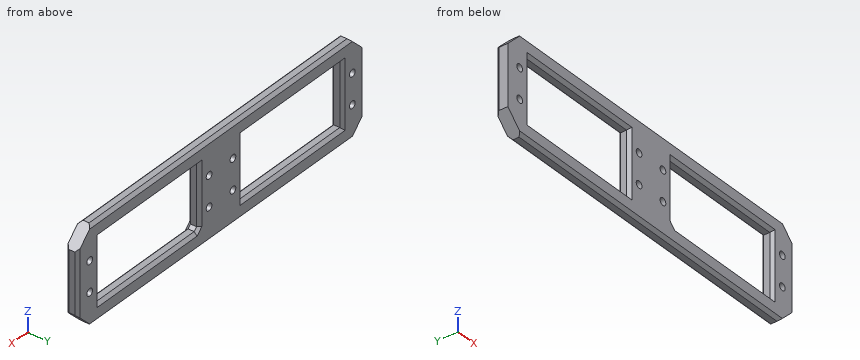
```python
from build123d import *

# Parameters (mm, degrees)
SKETCH1_W           = 120
SKETCH1_H           = 32
BOSS_EXTRUDE1_DEPTH = 4
SKETCH2_R           = 1.2
SKETCH2_W           = 42
SKETCH2_H           = 21
CUT_EXTRUDE1_DEPTH  = 4
CHAMFER1_SIZE       = 1
CUT_EXTRUDE2_DEPTH  = 10


with BuildPart() as part:
    # Sketch1 → Boss-Extrude1 (new body)
    with BuildSketch(Plane(origin=(0, 0, 0), x_dir=(1, 0, 0), z_dir=(0, 1, 0))):
        Rectangle(SKETCH1_W, SKETCH1_H)
    extrude(amount=BOSS_EXTRUDE1_DEPTH)

    # Sketch2 → Cut-Extrude1 (cut)
    with BuildSketch(Plane(origin=(0, 4, 0), x_dir=(1, 0, 0), z_dir=(0, 1, 0))):
        with Locations(Location((55, 5, 0), (0, 0, 270))):
            Circle(SKETCH2_R)
        with Locations(Location((55, -5, 0), (0, 0, 270))):
            Circle(SKETCH2_R)
        with Locations(Location((5, 5, 0), (0, 0, 270))):
            Circle(SKETCH2_R)
        with Locations(Location((5, -5, 0), (0, 0, 270))):
            Circle(SKETCH2_R)
        with Locations((30, 0)):
            Rectangle(SKETCH2_W, SKETCH2_H)
    cut_extrude1 = extrude(amount=-CUT_EXTRUDE1_DEPTH, mode=Mode.SUBTRACT)

    # Mirror1: Cut-Extrude1 across plane
    add(cut_extrude1.mirror(Plane(origin=(0, 0, 0), x_dir=(0, 0, 1), z_dir=(1, 0, 0))), mode=Mode.SUBTRACT)

    # Chamfer1
    chamfer1_edges = [part.edges().sort_by_distance(p)[0] for p in [
        (-60, 4, 0),
        (0, 4, 16),
        (9, 0, 0),
        (30, 0, -10.5),
        (9, 2, -10.5),
        (51, 0, 0),
        (30, 0, 10.5),
        (9, 4, 0),
        (30, 4, 10.5),
        (51, 4, 0),
        (30, 4, -10.5),
        (60, 4, 0),
        (0, 0, 16),
        (0, 0, -16),
        (60, 0, 0),
        (-9, 4, 0),
        (-30, 4, 10.5),
        (-51, 4, 0),
        (-30, 4, -10.5),
        (-9, 0, 0),
        (-30, 0, 10.5),
        (-51, 0, 0),
        (-30, 0, -10.5),
        (0, 4, -16),
        (60, 2, 16),
        (-60, 2, 16),
        (-60, 2, -16),
        (60, 2, -16),
    ]]
    chamfer(chamfer1_edges, length=CHAMFER1_SIZE)

    # Sketch3 → Cut-Extrude2 (cut)
    with BuildSketch(Plane.XZ):
        Polygon((-60, 10), (-54, 16), (-63.164716505, 19.318756061), align=None)
        Polygon((-60, -10), (-54, -16), (-62.553854867, -17.935195974), align=None)
    cut_extrude2 = extrude(amount=-CUT_EXTRUDE2_DEPTH, mode=Mode.SUBTRACT)

    # Mirror2: Cut-Extrude2 across plane
    add(cut_extrude2.mirror(Plane(origin=(0, 0, 0), x_dir=(0, 0, 1), z_dir=(1, 0, 0))), mode=Mode.SUBTRACT)


solid = part.part
```
Part model, mm, in its own coordinate system. Give positions to 0.01 mm unless a question says otherwise; leave off trailing zeros. Order: outer loops, then holes, each group sorted by start corner. A loop starts at its lowest first (then second) coordinate and runs counter-clockwise, first axis right, second up. Notation, with made-up numbers: M 68.5,46.5 L 78.5,46.5 A31 ccw 78.5,81.5 Z; hole C 71,-15.5 d5. An arc over 180 degrees is marked long. Use a Markdown table: item, result. Add a question column.
(1) Saw through at A-A, the plane x = 36. Give the cut face in (y, z).
(2) Probe line 1 along X through (y, z) = (1.85, 3); line 2 along Z through (x, y) = (-55, 2.9); line 3 along Z through (x, y) = (-5, 1). List the from-to ranges inside material, lowest first. Write a range as [from, to].
(3) Saw through at C-C, the plane y = 2.3. Give the number of separate pieces and of enclosed holes in the cut face, and give its area (3 significant figures).
(4) Saw through at B-B, the plane x = -5. Give the cut face in (y, z).
Answer key:
| question | item | result |
|---|---|---|
| 1 | outline | M 0,-15 L 1,-16 L 3,-16 L 4,-15 L 4,-11.5 L 3,-10.5 L 1,-10.5 L 0,-11.5 Z; M 0,11.5 L 1,10.5 L 3,10.5 L 4,11.5 L 4,15 L 3,16 L 1,16 L 0,15 Z |
| 2 | line 1 | [-60, -51], [-9, 9], [51, 60] |
| 2 | line 2 | [-15, -6.2], [-3.8, 3.8], [6.2, 15] |
| 2 | line 3 | [-16, -6.2], [-3.8, 3.8], [6.2, 16] |
| 3 | separate pieces | 1 |
| 3 | enclosed holes | 10 |
| 3 | area | 1,970 mm^2 |
| 4 | outline | M 0,-15 L 1,-16 L 3,-16 L 4,-15 L 4,-6.2 L 0,-6.2 Z; M 0,-3.8 L 4,-3.8 L 4,3.8 L 0,3.8 Z; M 0,6.2 L 4,6.2 L 4,15 L 3,16 L 1,16 L 0,15 Z |
